from build123d import *

# Parameters (mm, degrees)
F0_R       = 3.1
F0_R_2     = 25.2
F0_R_3     = 1.7
F1_DEPTH   = 3
F2_DEPTH   = 1
F0_R_4     = 3.2
F3_DEPTH   = 13
F0_R_5     = 1.4
F4_DEPTH   = 11.6
F5_DEPTH   = 0.6
F6_DEPTH   = 1
F7_SIZE2   = 0.8
F7_SIZE    = 1.4
F7_2_SIZE2 = 0.8
F7_2_SIZE  = 1.4
F7_3_SIZE2 = 0.8
F7_3_SIZE  = 1.4
F8_R       = 0.1
F9_SIZE    = 1.2


with BuildPart() as f1:
    # F0 (on Top) → F1 (new body)
    with BuildSketch(Plane.XY):
        Polygon((28.5, 16.4544826719), (28.5, 25.6920869789), (-28.5, 25.6920869789), (-28.5, 16.4544826719), (-36.5, 11.8356805184), (-8, -37.5277674973), (0, -32.9089653438), (8, -37.5277674973), (36.5, 11.8356805184), align=None)
        with Locations((0, -29.6)):
            Circle(F0_R, mode=Mode.SUBTRACT)
        Circle(F0_R_2, mode=Mode.SUBTRACT)
        with Locations((-25.634351952, 14.8)):
            Circle(F0_R, mode=Mode.SUBTRACT)
        with Locations((25.634351952, 14.8)):
            Circle(F0_R, mode=Mode.SUBTRACT)
        with Locations((-25.634351952, 14.8)):
            Circle(F0_R)
        with Locations((-25.634351952, 14.8)):
            Circle(F0_R_3, mode=Mode.SUBTRACT)
        with Locations((25.634351952, 14.8)):
            Circle(F0_R)
        with Locations((25.634351952, 14.8)):
            Circle(F0_R_3, mode=Mode.SUBTRACT)
        with Locations((0, -29.6)):
            Circle(F0_R)
        with Locations((0, -29.6)):
            Circle(F0_R_3, mode=Mode.SUBTRACT)
        Polygon((-28.5, 16.4544826719), (-28.5, 25.6920869789), (-28.981864252, 25.6920869789), (-28.981864252, 16.7326871275), (-36.740932126, 12.2529872018), (-36.5, 11.8356805184), align=None)
        Polygon((28.981864252, 25.6920869789), (28.5, 25.6920869789), (28.5, 16.4544826719), (36.5, 11.8356805184), (36.740932126, 12.2529872018), (28.981864252, 16.7326871275), align=None)
        Polygon((7.759067874, -37.9450741808), (8, -37.5277674973), (0, -32.9089653438), (-8, -37.5277674973), (-7.759067874, -37.9450741808), (0, -33.4653742551), align=None)
    extrude(amount=F1_DEPTH)

    # F0 (on Top) → F2 (join)
    with BuildSketch(Plane.XY):
        Circle(F0_R_2)
        with BuildLine():
            ThreePointArc((19.3997487421, 12.3551506969), (19.918584287, 11.5), (20.3997487421, 10.6230998893))
            ThreePointArc((20.3997487421, 10.6230998893), (22.3404814302, 5.468353451), (23, 0))
            ThreePointArc((23, 0), (16.6132477258, -15.9059737206), (1, -22.9782505862))
            ThreePointArc((1, -22.9782505862), (0, -23), (-1, -22.9782505862))
            ThreePointArc((-1, -22.9782505862), (-19.918584287, -11.5), (-20.3997487421, 10.6230998893))
            ThreePointArc((-20.3997487421, 10.6230998893), (-19.918584287, 11.5), (-19.3997487421, 12.3551506969))
            ThreePointArc((-19.3997487421, 12.3551506969), (0, 23), (19.3997487421, 12.3551506969))
        make_face(mode=Mode.SUBTRACT)
        with BuildLine():
            Line((1, -22.9782505862), (0.2000154666, -4.9959977795))
            ThreePointArc((0.2000154666, -4.9959977795), (0, -5), (-0.2000154666, -4.9959977795))
            Line((-0.2000154666, -4.9959977795), (-1, -22.9782505862))
            ThreePointArc((-1, -22.9782505862), (0, -23), (1, -22.9782505862))
        make_face()
        with BuildLine():
            ThreePointArc((4.226653261, 2.671217365), (4.3301270189, 2.5), (4.4266687276, 2.3247804145))
            Line((4.4266687276, 2.3247804145), (20.3997487421, 10.6230998893))
            ThreePointArc((20.3997487421, 10.6230998893), (19.918584287, 11.5), (19.3997487421, 12.3551506969))
            Line((19.3997487421, 12.3551506969), (4.226653261, 2.671217365))
        make_face()
        with BuildLine():
            ThreePointArc((-4.4266687276, 2.3247804145), (-4.3301270189, 2.5), (-4.226653261, 2.671217365))
            Line((-4.226653261, 2.671217365), (-19.3997487421, 12.3551506969))
            ThreePointArc((-19.3997487421, 12.3551506969), (-19.918584287, 11.5), (-20.3997487421, 10.6230998893))
            Line((-20.3997487421, 10.6230998893), (-4.4266687276, 2.3247804145))
        make_face()
        with BuildLine():
            Line((-0.2000154666, -4.9959977795), (-0.1555714282, -3.9969735464))
            ThreePointArc((-0.1555714282, -3.9969735464), (-3.4641016151, -2), (-3.5392663435, 1.8637579643))
            Line((-3.5392663435, 1.8637579643), (-4.4266687276, 2.3247804145))
            ThreePointArc((-4.4266687276, 2.3247804145), (-4.3301270189, -2.5), (-0.2000154666, -4.9959977795))
        make_face()
        with BuildLine():
            ThreePointArc((3.5392663435, 1.8637579643), (3.883108637, 0.9599308897), (4, 0))
            ThreePointArc((4, 0), (2.8829052805, -2.7728788548), (0.1555714282, -3.9969735464))
            Line((0.1555714282, -3.9969735464), (0.2000154666, -4.9959977795))
            ThreePointArc((0.2000154666, -4.9959977795), (3.6055566375, -3.4640960341), (5, 0))
            ThreePointArc((5, 0), (4.8545516599, 1.1972168479), (4.4266687276, 2.3247804145))
            Line((4.4266687276, 2.3247804145), (3.5392663435, 1.8637579643))
        make_face()
        with BuildLine():
            ThreePointArc((-3.3836949154, 2.1332155821), (0, 4), (3.3836949154, 2.1332155821))
            Line((3.3836949154, 2.1332155821), (4.226653261, 2.671217365))
            ThreePointArc((4.226653261, 2.671217365), (0, 5), (-4.226653261, 2.671217365))
            Line((-4.226653261, 2.671217365), (-3.3836949154, 2.1332155821))
        make_face()
        with BuildLine():
            Line((0.4330127019, 0.25), (3.5392663435, 1.8637579643))
            ThreePointArc((3.5392663435, 1.8637579643), (3.4641016151, 2), (3.3836949154, 2.1332155821))
            Line((3.3836949154, 2.1332155821), (0.4330127019, 0.25))
        make_face()
        with BuildLine():
            Line((-0.4330127019, 0.25), (-3.3836949154, 2.1332155821))
            ThreePointArc((-3.3836949154, 2.1332155821), (-3.4641016151, 2), (-3.5392663435, 1.8637579643))
            Line((-3.5392663435, 1.8637579643), (-0.4330127019, 0.25))
        make_face()
        with BuildLine():
            ThreePointArc((-0.1555714282, -3.9969735464), (0, -4), (0.1555714282, -3.9969735464))
            Line((0.1555714282, -3.9969735464), (0, -0.5))
            Line((0, -0.5), (-0.1555714282, -3.9969735464))
        make_face()
        with BuildLine():
            Line((0.2000154666, -4.9959977795), (0.1555714282, -3.9969735464))
            ThreePointArc((0.1555714282, -3.9969735464), (0, -4), (-0.1555714282, -3.9969735464))
            Line((-0.1555714282, -3.9969735464), (-0.2000154666, -4.9959977795))
            ThreePointArc((-0.2000154666, -4.9959977795), (0, -5), (0.2000154666, -4.9959977795))
        make_face()
        with BuildLine():
            ThreePointArc((3.3836949154, 2.1332155821), (3.4641016151, 2), (3.5392663435, 1.8637579643))
            Line((3.5392663435, 1.8637579643), (4.4266687276, 2.3247804145))
            ThreePointArc((4.4266687276, 2.3247804145), (4.3301270189, 2.5), (4.226653261, 2.671217365))
            Line((4.226653261, 2.671217365), (3.3836949154, 2.1332155821))
        make_face()
        with BuildLine():
            ThreePointArc((-3.5392663435, 1.8637579643), (-3.4641016151, 2), (-3.3836949154, 2.1332155821))
            Line((-3.3836949154, 2.1332155821), (-4.226653261, 2.671217365))
            ThreePointArc((-4.226653261, 2.671217365), (-4.3301270189, 2.5), (-4.4266687276, 2.3247804145))
            Line((-4.4266687276, 2.3247804145), (-3.5392663435, 1.8637579643))
        make_face()
    extrude(amount=F2_DEPTH)

    # F0 (on Top) → F3 (join)
    with BuildSketch(Plane.XY):
        Polygon((-28.981864252, 16.7326871275), (-28.981864252, 25.6920869789), (-32.9199963413, 25.6920869789), (-38.7099981707, 15.6635096346), (-36.740932126, 12.2529872018), align=None)
        with Locations((-32.5625551823, 18.8)):
            Circle(F0_R_4, mode=Mode.SUBTRACT)
        Polygon((5.7900018293, -41.3555966135), (7.759067874, -37.9450741808), (0, -33.4653742551), (-7.759067874, -37.9450741808), (-5.7900018293, -41.3555966135), align=None)
        with Locations((0, -37.6)):
            Circle(F0_R_4, mode=Mode.SUBTRACT)
        Polygon((32.9199963413, 25.6920869789), (28.981864252, 25.6920869789), (28.981864252, 16.7326871275), (36.740932126, 12.2529872018), (38.7099981707, 15.6635096346), align=None)
        with Locations((32.5625551823, 18.8)):
            Circle(F0_R_4, mode=Mode.SUBTRACT)
    extrude(amount=F3_DEPTH)

    # F0 (on Top) → F4 (join)
    with BuildSketch(Plane.XY):
        with Locations((0, -37.6)):
            Circle(F0_R_4)
        with Locations((0, -37.6)):
            Circle(F0_R_5, mode=Mode.SUBTRACT)
        with Locations((-32.5625551823, 18.8)):
            Circle(F0_R_4)
        with Locations((-32.5625551823, 18.8)):
            Circle(F0_R_5, mode=Mode.SUBTRACT)
        with Locations((32.5625551823, 18.8)):
            Circle(F0_R_4)
        with Locations((32.5625551823, 18.8)):
            Circle(F0_R_5, mode=Mode.SUBTRACT)
    extrude(amount=F4_DEPTH)

    # F0 (on Top) → F5 (join)
    with BuildSketch(Plane.XY):
        with Locations((0, -37.6)):
            Circle(F0_R_5)
        with Locations((-32.5625551823, 18.8)):
            Circle(F0_R_5)
        with Locations((32.5625551823, 18.8)):
            Circle(F0_R_5)
    extrude(amount=F5_DEPTH)

    # F0 (on Top) → F6 (cut)
    with BuildSketch(Plane.XY):
        with Locations((25.634351952, 14.8)):
            Circle(F0_R)
        with Locations((25.634351952, 14.8)):
            Circle(F0_R_3, mode=Mode.SUBTRACT)
        with Locations((-25.634351952, 14.8)):
            Circle(F0_R)
        with Locations((-25.634351952, 14.8)):
            Circle(F0_R_3, mode=Mode.SUBTRACT)
        with Locations((0, -29.6)):
            Circle(F0_R)
        with Locations((0, -29.6)):
            Circle(F0_R_3, mode=Mode.SUBTRACT)
    extrude(amount=F6_DEPTH, mode=Mode.SUBTRACT)

    # F7
    f7_edges = [f1.edges().sort_by_distance(p)[0] for p in [
        (-33.962555, 18.8, 11.6),
    ]]
    f7_side = f1.faces().sort_by_distance((-33.962555, 18.8, 6.1))[0]
    chamfer(f7_edges, length=F7_SIZE, length2=F7_SIZE2, reference=f7_side)

    # F7#2
    f7_2_edges = [f1.edges().sort_by_distance(p)[0] for p in [
        (31.162555, 18.8, 11.6),
    ]]
    f7_2_side = f1.faces().sort_by_distance((31.162555, 18.8, 6.1))[0]
    chamfer(f7_2_edges, length=F7_2_SIZE, length2=F7_2_SIZE2, reference=f7_2_side)

    # F7#3
    f7_3_edges = [f1.edges().sort_by_distance(p)[0] for p in [
        (-1.4, -37.6, 11.6),
    ]]
    f7_3_side = f1.faces().sort_by_distance((-1.4, -37.6, 6.1))[0]
    chamfer(f7_3_edges, length=F7_3_SIZE, length2=F7_3_SIZE2, reference=f7_3_side)

    # F8
    f8_edges = [f1.edges().sort_by_distance(p)[0] for p in [
        (-0.433013, 0.25, 0.5),
        (0.433013, 0.25, 0.5),
        (0, -0.5, 0.5),
    ]]
    fillet(f8_edges, radius=F8_R)

    # F9
    f9_edges = [f1.edges().sort_by_distance(p)[0] for p in [
        (-22.25, -12.846043, 0),
        (-35.814997, 20.677798, 0),
        (0, 25.692087, 0),
        (35.814997, 20.677798, 0),
        (22.25, -12.846043, 0),
        (0, -41.355597, 0),
    ]]
    chamfer(f9_edges, length=F9_SIZE)


solid = f1.part
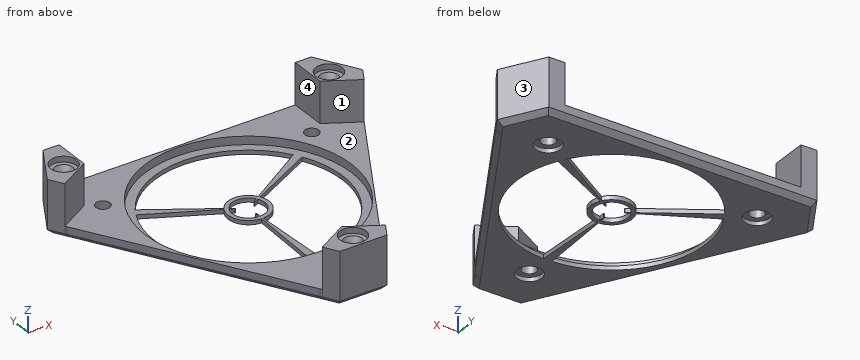
Source: CAD feature listing. Evaluate the final solid. Frame: model axes, mm. Face numbers are marked on the shaded views. A direction names the side the tool comes from. Give positions to 0.01 mm unless a question says otherwise; leave off trailing zeros. Order: outer loops, then holes, each group sorted by start corner. A loop starts at its lowest first (then second) coordinate and runs counter-clockwise, first axis right, second up. Notation, with made-up numbers: (23, -16.75) -> (81, -16.75) arc R18 ccw to (81, -7.75) -> close; hole circle Ø3 at (22, 12.25). An arc over 180 degrees is marked (long way). Use a Markdown table: item, result.
1) Section query A-A, the plane z = 7.75. Return the cut outline in (x, y), then the cut area to 3 significant figures.
Answer list:
| item | result |
|---|---|
| outline | (-38.71, 15.66) -> (-36.74, 12.25) -> (-28.98, 16.73) -> (-28.98, 25.69) -> (-32.92, 25.69) -> close; (-7.76, -37.95) -> (-5.79, -41.36) -> (5.79, -41.36) -> (7.76, -37.95) -> (0, -33.47) -> close; (28.98, 16.73) -> (36.74, 12.25) -> (38.71, 15.66) -> (32.92, 25.69) -> (28.98, 25.69) -> close; hole circle Ø2.8 at (-32.56, 18.8); hole circle Ø2.8 at (0, -37.6); hole circle Ø2.8 at (32.56, 18.8) |
| area | 224 mm² |
2) Section query C-C, the plane y = -13. Return the cut outline in (x, z).
Answer list:
| item | result |
|---|---|
| outline | (-22.16, 1.2) -> (-20.78, 0) -> (-18.97, 0) -> (-18.97, 1) -> (-21.59, 1) -> (-21.59, 3) -> (-22.16, 3) -> close; (-0.56, 0) -> (0.56, 0) -> (0.56, 1) -> (-0.56, 1) -> close; (18.97, 0) -> (20.78, 0) -> (22.16, 1.2) -> (22.16, 3) -> (21.59, 3) -> (21.59, 1) -> (18.97, 1) -> close |
3) Contact query for flat-ended pins moving along their axis: P1, Ø10, axis at x = 0, y = -29.6, coming from the +Z side; P2, Ø1.4, axis at x = 33, y = 18, coming from the +Z side; P3, Ø2, axis at x = -33, y = 18.5, coming from the +Z side; P4, Ø3, axis at x = 0, y = -38, coming from the +Z side (3 decimals). Output: stop coordinate, or through.
Answer list:
| item | result |
|---|---|
| P1 | z = 13 |
| P2 | z = 10.57 |
| P3 | z = 10.43 |
| P4 | z = 11.075 |
4) Reachability of the marked faces 1, 2, 3 and 4 from +Z, -Z, +X, -X, +Y, -Y: full face, straight path, thin tool, end or side. Return the list, or none.
Answer list:
| item | result |
|---|---|
| face 1 | +Z, -Y |
| face 2 | +Z |
| face 3 | +Z, -Z, +X, +Y |
| face 4 | +Z, +Y, -Y |
5) Section query B-B, the plane y = -29.6. Return the cut outline in (x, z), then the cut area to 3 significant figures.
Answer list:
| item | result |
|---|---|
| outline | (-12.58, 1.2) -> (-11.19, 0) -> (-3.1, 0) -> (-3.1, 1) -> (-1.7, 1) -> (-1.7, 3) -> (-12.58, 3) -> close; (1.7, 1) -> (3.1, 1) -> (3.1, 0) -> (11.19, 0) -> (12.58, 1.2) -> (12.58, 3) -> (1.7, 3) -> close |
| area | 60.8 mm² |
6) Ray query, line 1 along Y through (x, z) = (0, 1.75); line 2 along Z through (x, y) = (30, 14); line 3 along Z through (x, y) = (-16, -17). Return the intervals inside material, ascending. Write a range as [from, to].
Answer list:
| item | result |
|---|---|
| line 1 | [-41.36, -39], [-36.2, -31.3], [-27.9, -25.2], [25.2, 25.69] |
| line 2 | [0, 3] |
| line 3 | [0, 1] |
